Check sheet for the drawn part. Datum: minimum x, y, z corner. Units: mm. A direction names the side the tool comes from. Round coordinates to 2 decimals unless told otherwise and drop trailing zeros. Write each loop counter-clockwise with the first axis right and the second up, starting at its lowest first coordinate (ties: lowest second). Pieces come first, ordered by that corner, then holes. Notation, with made-up numbers: (61.5, 84) - (103.5, 84) arc R20 cw to (103.5, 113) - close; hole circle Ø1 at (40, 81). An arc over 180 degrees is marked (long way). Answer as a JSON object with one key per item and string values.
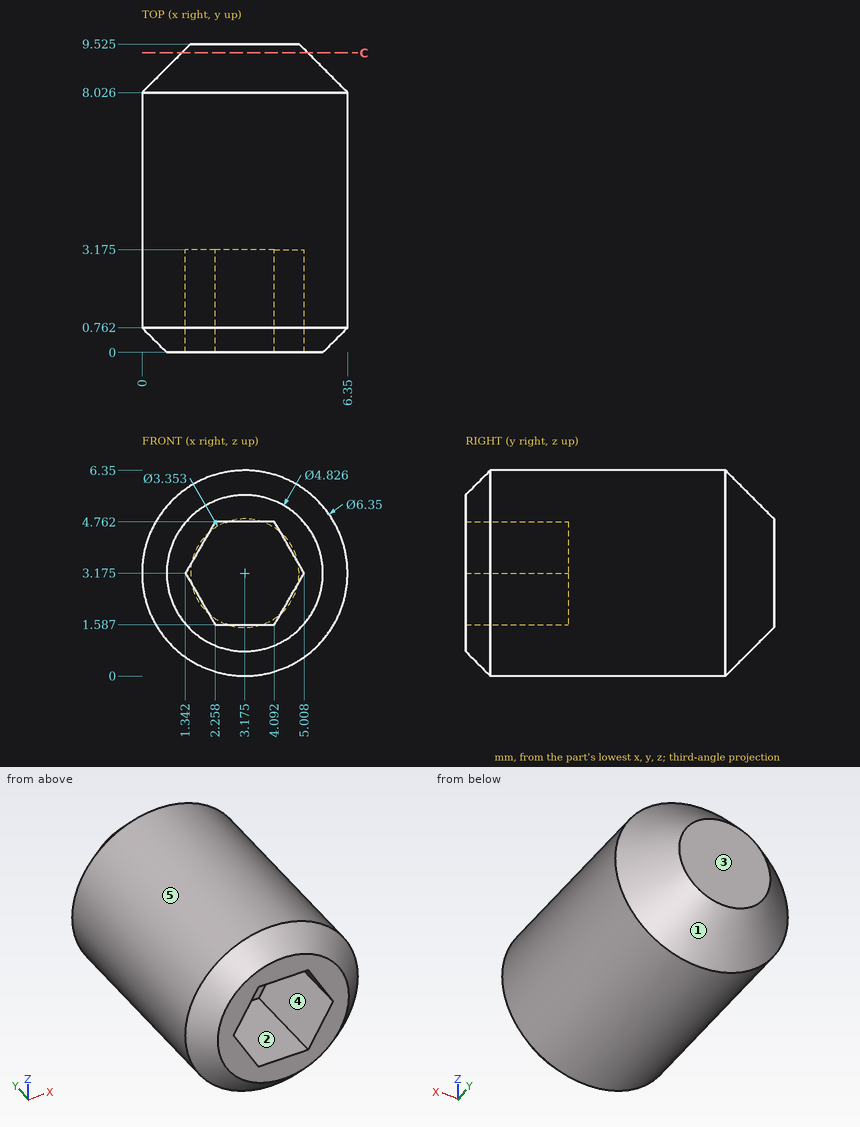
1. Access from +Z, -Z, +X, -X, +Y, -Y to the whole of each face (thin tool, end or side, straight path). Record for the marked faces 1 and 2.
Completed:
{"face 1": "+Y", "face 2": "-Y"}
2. Cross-section at C-C (y = 9.25). Record the boundary of the cut face in (x, z) (1 decimal).
Completed:
{"outline": "circle Ø3.9 at (3.2, 3.2)"}
3. Mould release check, pull along X, two halves, no side actions. Record for the marked faces 3, 4 and 5: released by +X, released by -X, zero draft, split by the parting line, or undercut.
Completed:
{"face 3": "zero draft", "face 4": "undercut", "face 5": "split by the parting line"}
4. Go/stop test with flat-tipped pins: pin 1 (1 mm diameter, centred on x = 4.5, y = 5.5, fed in from +Z); pin 2 (1 mm diameter, centred on x = 1, y = 5, fed in from -Z). Record where each tip stops, or that it passes through.
Completed:
{"pin 1": "stops at z = 6.24", "pin 2": "stops at z = 0.48"}
5. Material ranges on probe 1 along Z at (x, y) = (4, 2.25); probe 2 along X at (y, z) = (2.5, 3) (1 decimal); probe 3 along Y at (x, z) = (1.75, 4.25) (1 decimal), recorded low to high. Write a range as from..to.
Completed:
{"probe 1": "z = 0.11..1.59, 4.76..6.24", "probe 2": "x = 0..1.4, 4.9..6.3", "probe 3": "y = 0..9.4"}
